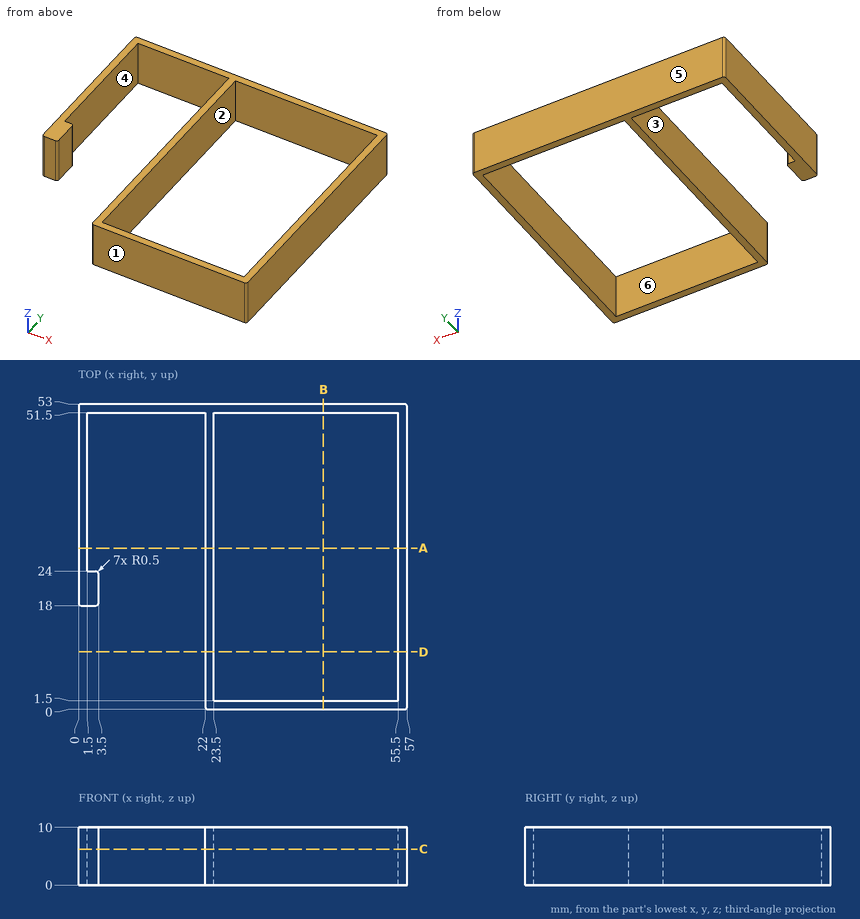
Geometry: see drawing. Coordinates: mm, zero at the bounding-box minimum. A direction names the side the tool comes from. Give positions to 0.01 mm unless a question says otherwise; leave off trailing zeros. Loops run counter-clockwise (first coordinate to the right, second up) from the corner with the lowest first, then second, coordinate; pieces in that order, holes last. Notation, with made-up numbers: (64.25, 6.25) -> (97.25, 6.25) arc R15 cw to (97.25, 16.25) -> close; hole circle Ø7 at (69.5, 3). An arc over 180 degrees is marked (long way). Answer as a JSON object with one key per item and string values. Group by question number.
Item 1: Pull-direction query (Y, two-part tool) for the marked faces 3, 4, 5 and 6; classes: released by +Y, released by -Y, zero draft, split by the parting line, or undercut.
Item 2: Reachability of the marked faces 1 and 2 from +Z, -Z, +X, -X, +Y, -Y: full face, straight path, thin tool, end or side. Return the list, or none.
Item 3: Pin query (flat end, axial travel): P1, Ø3, axis at y = 35, z = 4.5, coming from the -X side; P2, Ø1.2, axis at x = 2, z = 2.5, coming from the -Y side. Return the tip coordinate at first contact, or that it passes through.
Item 4: Cut plane D-D, the plane y = 10. Return the cut outline in (x, z), and give its area (3 significant figures).
Item 5: Line query: probe 1 along X at (y, z) = (45.5, 4); probe 2 along X at (y, z) = (23.5, 6.5); probe 3 along X at (y, z) = (16.5, 3.25). Output: solid intervals per line, ascending.
Item 6: Cut plane A-A, the plane y = 28. Return the cut outline in (x, z), and give its area (3 significant figures).
Item 7: Cut plane B-B, the plane x = 42.5. Return the cut outline in (y, z), and give its area (3 significant figures).
Item 8: Cut plane C-C, the plane z = 6.25. Return the cut outline in (x, y).
Checks:
{
 "1": {"face 3": "zero draft", "face 4": "undercut", "face 5": "released by +Y", "face 6": "undercut"},
 "2": {"face 1": "+Z, -Z, +X, -X, -Y", "face 2": "+Z, -Z"},
 "3": {"P1": "stops at x = 0", "P2": "stops at y = 18"},
 "4": {"outline": "(22, 0) -> (23.5, 0) -> (23.5, 10) -> (22, 10) -> close; (55.5, 0) -> (57, 0) -> (57, 10) -> (55.5, 10) -> close", "area": "30.0 mm²"},
 "5": {"probe 1": "x = 0 to 1.5, 22 to 23.5, 55.5 to 57", "probe 2": "x = 0 to 3.5, 22 to 23.5, 55.5 to 57", "probe 3": "x = 22 to 23.5, 55.5 to 57"},
 "6": {"outline": "(0, 0) -> (1.5, 0) -> (1.5, 10) -> (0, 10) -> close; (22, 0) -> (23.5, 0) -> (23.5, 10) -> (22, 10) -> close; (55.5, 0) -> (57, 0) -> (57, 10) -> (55.5, 10) -> close", "area": "45.0 mm²"},
 "7": {"outline": "(0, 0) -> (1.5, 0) -> (1.5, 10) -> (0, 10) -> close; (51.5, 0) -> (53, 0) -> (53, 10) -> (51.5, 10) -> close", "area": "30.0 mm²"},
 "8": {"outline": "(0, 18.5) arc R0.5 ccw to (0.5, 18) -> (3, 18) arc R0.5 ccw to (3.5, 18.5) -> (3.5, 23.5) arc R0.5 ccw to (3, 24) -> (1.5, 24) -> (1.5, 51.5) -> (22, 51.5) -> (22, 0.5) arc R0.5 ccw to (22.5, 0) -> (56.5, 0) arc R0.5 ccw to (57, 0.5) -> (57, 52.5) arc R0.5 ccw to (56.5, 53) -> (0.5, 53) arc R0.5 ccw to (0, 52.5) -> close; hole (23.5, 1.5) -> (55.5, 1.5) -> (55.5, 51.5) -> (23.5, 51.5) -> close"}
}
